Part model, mm, in its own coordinate system. Face numbers are marked on the shaded views. A direction names the side the tool comes from. Give positions to 0.01 mm unless a question says otherwise; leave off trailing zeros. Order: outer loops, then holes, each group sorted by start corner. A loop starts at its lowest first (then second) coordinate and runs counter-clockwise, first axis right, second up.
1. Slice it at A-A on x = 0. List the corners of the cut face in (y, z), and give its area (3 significant figures).
2. Drop flat-ended pins along their axis: pin 1 Ø17 at (y, z) = (-1.5, 69) entering from +X; pin 2 Ø5 at (y, z) = (8, 47) entering from +X; pin 3 Ø6 at (y, z) = (0, 42) entering from +X. Give the stop position or say it passes through.
3. Slice it at C-C on y = 30. List the corners of the cut face in (x, z).
4. Slice it at D-D on z = 17.5. List the corners of the cut face in (x, y), and give its area (3 significant figures).
5. Slice it at B-B on z = 67. List the corners of the cut face in (x, y).
6. Probe line 1 (Z direction, x = 15.5, y = -36.5); line 2 (X direction, y = -1, z = 6.5); line 3 (Y direction, x = -16.5, z = 54.5). List the from-to ranges inside material, lowest first.
7. Mould opens along Y. For the marked faces 3 and 4 say: +Y half, -Y half, draft (parallel to the pull), parting line (faces both ways), or undercut.
8. Which spindle directions (+Z, -Z, +X, -X, +Y, -Y) get a long thin tool onto all of the face, cutting with end or side? Do the marked faces 1 and 2. Say none if no direction does.
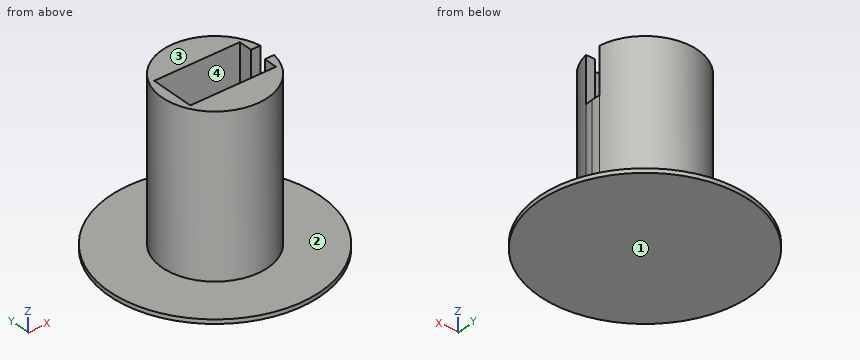
from build123d import *

# Parameters (mm, degrees)
SKETCH1_R           = 50
BOSS_EXTRUDE1_DEPTH = 2
SKETCH1_3_W         = 4.75
SKETCH1_3_H         = 8
BOSS_EXTRUDE2_DEPTH = 50
BOSS_EXTRUDE3_DEPTH = 77
BOSS_EXTRUDE7_DEPTH = 55


with BuildPart() as part:
    # Sketch1 → Boss-Extrude1 (new body)
    # profile 1 of 3: a face of its own
    with BuildSketch(Plane.XY):
        Circle(SKETCH1_R)
        with BuildLine():
            ThreePointArc((24.677925359, -4), (-25, 0), (24.677925359, 4))
            Line((24.677925359, 4), (25, 4))
            Line((25, 4), (25, 0))
            Line((25, 0), (25, -4))
            Line((25, -4), (24.677925359, -4))
        make_face(mode=Mode.SUBTRACT)
    # profile 2 of 3: a face of its own
    with BuildSketch(Plane.XY):
        with BuildLine():
            ThreePointArc((25, 0), (24.919351255, -2.00647278), (24.677925359, -4))
            Line((24.677925359, -4), (25, -4))
            Line((25, -4), (25, 0))
        make_face()
    # profile 3 of 3: a face of its own
    with BuildSketch(Plane.XY):
        with BuildLine():
            Line((25, 4), (24.677925359, 4))
            ThreePointArc((24.677925359, 4), (24.919351255, 2.00647278), (25, 0))
            Line((25, 0), (25, 4))
        make_face()
    extrude(amount=BOSS_EXTRUDE1_DEPTH)



with BuildPart() as body_2:
    # Sketch1_3 → Boss-Extrude2 (new body)
    with BuildSketch(Plane.XY):
        Polygon((20.25, 10.5), (-20.25, 10.5), (-20.25, -10.5), (20.25, -10.5), (20.25, -4), (15.5, -4), (15.5, 4), (20.25, 4), align=None)
        with Locations((17.875, 0)):
            Rectangle(SKETCH1_3_W, SKETCH1_3_H)
    extrude(amount=BOSS_EXTRUDE2_DEPTH)


with BuildPart() as part_1:
    add(part.part)

    add(body_2.part)  # Boss-Extrude3 merges body 2
    # Sketch1_4 → Boss-Extrude3 (add)
    with BuildSketch(Plane.XY):
        with BuildLine():
            Line((-20.25, -10.5), (-20.25, 10.5))
            Line((-20.25, 10.5), (20.25, 10.5))
            Line((20.25, 10.5), (20.25, 4))
            Line((20.25, 4), (24.677925359, 4))
            ThreePointArc((24.677925359, 4), (-25, 0), (24.677925359, -4))
            Line((24.677925359, -4), (20.25, -4))
            Line((20.25, -4), (20.25, -10.5))
            Line((20.25, -10.5), (-20.25, -10.5))
        make_face()
    extrude(amount=BOSS_EXTRUDE3_DEPTH)

    # Sketch1_7 → Boss-Extrude7 (add)
    with BuildSketch(Plane.XY):
        with BuildLine():
            Line((24.677925359, 4), (20.25, 4))
            Line((20.25, 4), (20.25, -4))
            Line((20.25, -4), (24.677925359, -4))
            ThreePointArc((24.677925359, -4), (24.919351255, -2.00647278), (25, 0))
            ThreePointArc((25, 0), (24.919351255, 2.00647278), (24.677925359, 4))
        make_face()
    extrude(amount=BOSS_EXTRUDE7_DEPTH)


solid = part_1.part
Data:
1. outline: (-50, 0) - (50, 0) - (50, 2) - (25, 2) - (25, 77) - (10.5, 77) - (10.5, 50) - (-10.5, 50) - (-10.5, 77) - (-25, 77) - (-25, 2) - (-50, 2) - close
1. area: 3,380 mm2
2. pin 1: stops at x = 24.68
2. pin 2: stops at x = 24.39
2. pin 3: stops at x = 25
3. outline: (-40, 0) - (40, 0) - (40, 2) - (-40, 2) - close
4. outline: circle Ø50 at (0, 0)
4. area: 1,960 mm2
5. outline: (-20.25, -10.5) - (-20.25, 10.5) - (20.25, 10.5) - (20.25, 4) - (24.68, 4) arc R25 ccw (long way) to (24.68, -4) - (20.25, -4) - (20.25, -10.5) - close
6. line 1: z = 0 to 2
6. line 2: x = -24.98 to 24.98
6. line 3: y = -18.78 to -10.5, 10.5 to 18.78
7. face 3: draft
7. face 4: undercut
8. face 1: -Z, +X, -X, +Y, -Y
8. face 2: +Z
